Part model, mm, in its own coordinate system. A direction names the side the tool comes from. Round coordinates to 2 decimals unless told otherwise and drop trailing zeros. Loops run counter-clockwise (first coordinate to the right, second up) from the corner with the lowest first, then second, coordinate; pieces in that order, holes last. Notation, with made-up numbers: (53, -17.75) -> (109, -17.75) arc R13 ccw to (109, -6.75) -> close; hole circle Ø1 at (7, 76.25). An arc over 180 degrees is marked (long way). Use a Markdown table: item, result. Add a question column.
Item 1: Cut at A-A, the plane x = -10.5. List the corners of the cut face in (y, z), plus the area to 4 significant figures.
Item 2: Flat gauge pins, fed straight in: pin 1 (8 mm diameter, centred on x = -3.5, y = 23.5, fed in from -Z); pin 2 (0.6 mm diameter, centred on y = 13.5, z = 0.5, fed in from -X); pin 3 (6.5 mm diameter, centred on x = 16.5, y = -21.5, fed in from -Z). Where does each tip first touch, or does it go through?
Item 3: Two-plate mould, pull along Y, no slides. Class faces 4 (the face through (1, 49.682, -28)), 5 (the face through (48.16, -21.99, -3.94)), 6 (the face through (17, -22, -8)): pulls with the +Y half, pulls with the -Y half, needs draft (parallel to the pull), parting line crosses it, or undercut.
Item 4: Cut at B-B, the plane y = 37.5. List the corners of the cut face in (x, z), plus the area to 3 significant figures.
Item 5: Cut at C-C, the plane z = -2.5. List the corners of the cut face in (x, y).
Item 6: Which spindle directions (+Z, -Z, +X, -X, +Y, -Y) get a long thin tool onto all of the face, cutting with end or side? Do faces 1 (the face through (52, -22, -8)), 2 (the face through (1, 5, 2.54)), 3 (the face through (17.77, -24.39, -3.94)). Say none if no direction does.
Item 7: Cut at D-D, the plane x = 46.5. List the corners of the cut face in (y, z), plus the area to 3 significant figures.
Item 8: Probe line 1 (Y direction, x = -48, z = -0.5); line 2 (Z direction, x = 71, y = 17.5); line 3 (Z direction, x = 49, y = -20.5). List the from-to ranges inside material, lowest first. Write a range as [from, to].
```python
from build123d import *

# Parameters (mm, degrees)
SKETCH1_W           = 150
SKETCH1_H           = 85
BOSS_EXTRUDE1_DEPTH = 2.54
SKETCH2_W           = 20
SKETCH2_H           = 20
CUT_EXTRUDE1_DEPTH  = 2.54
SKETCH3_R           = 3
BOSS_EXTRUDE2_DEPTH = 8
SKETCH9_R           = 0.5
CUT_EXTRUDE7_DEPTH  = 4
CUT_EXTRUDE8_DEPTH  = 85
SKETCH11_W          = 150
SKETCH11_H          = 60
BOSS_EXTRUDE3_DEPTH = 2.54


with BuildPart() as part:
    # Sketch1 → Boss-Extrude1 (new body)
    with BuildSketch(Plane.XY):
        with Locations((2.158007809, 4.641833841)):
            Rectangle(SKETCH1_W, SKETCH1_H)
    extrude(amount=BOSS_EXTRUDE1_DEPTH)

    # Sketch2 → Cut-Extrude1 (cut)
    with BuildSketch(Plane(origin=(0, 0, 0), x_dir=(-1, 0, 0), z_dir=(0, 0, -1))):
        with Locations((7.841992191, -13.158166159)):
            Rectangle(SKETCH2_W, SKETCH2_H)
    extrude(amount=-CUT_EXTRUDE1_DEPTH, mode=Mode.SUBTRACT)

    # Sketch3 → Boss-Extrude2 (add)
    with BuildSketch(Plane(origin=(0, 0, 0), x_dir=(-1, 0, 0), z_dir=(0, 0, -1))):
        with Locations(Location((-51.158007809, -21.858166159, 0), (0, 0, 180))):
            Circle(SKETCH3_R)
        with Locations(Location((-16.158007809, -21.858166159, 0), (0, 0, 180))):
            Circle(SKETCH3_R)
    extrude(amount=BOSS_EXTRUDE2_DEPTH)

    # Sketch9 → Cut-Extrude7 (cut)
    with BuildSketch(Plane(origin=(0, 0, -8), x_dir=(-1, 0, 0), z_dir=(0, 0, -1))):
        with Locations((-51.158007809, -21.858166159)):
            Circle(SKETCH9_R)
        with Locations((-16.158007809, -21.858166159)):
            Circle(SKETCH9_R)
    extrude(amount=-CUT_EXTRUDE7_DEPTH, mode=Mode.SUBTRACT)

    # Sketch10 → Cut-Extrude8 (cut)
    with BuildSketch(Plane(origin=(0, 47.141833841, 0), x_dir=(1, 0, 0), z_dir=(0, 1, 0))):
        Polygon((-69.666992191, -1.27), (-69.666992191, -2.54), (-72.841992191, -2.54), (-72.841992191, 0), (-70.936992191, 0), (-70.936992191, -1.27), align=None)
        Polygon((75.888007809, 0), (75.888007809, -1.27), (74.618007809, -1.27), (74.618007809, -2.54), (77.158007809, -2.54), (77.158007809, 0), align=None)
    extrude(amount=-CUT_EXTRUDE8_DEPTH, mode=Mode.SUBTRACT)

    # Sketch11 → Boss-Extrude3 (add)
    with BuildSketch(Plane(origin=(0, 47.141833841, 0), x_dir=(1, 0, 0), z_dir=(0, 1, 0))):
        with Locations((2.158007809, 27.46)):
            Rectangle(SKETCH11_W, SKETCH11_H)
    extrude(amount=BOSS_EXTRUDE3_DEPTH)


solid = part.part
```
A:
| question | item | result |
|---|---|---|
| 1 | outline | (-37.86, 0) -> (-23.16, 0) -> (-23.16, 2.54) -> (-37.86, 2.54) -> close; (-3.16, 0) -> (47.14, 0) -> (47.14, -57.46) -> (49.68, -57.46) -> (49.68, 2.54) -> (-3.16, 2.54) -> close |
| 1 | area | 317.5 mm^2 |
| 2 | pin 1 | stops at z = 0 |
| 2 | pin 2 | stops at x = -70.94 |
| 2 | pin 3 | stops at z = -8 |
| 3 | face 4 | pulls with the +Y half |
| 3 | face 5 | undercut |
| 3 | face 6 | needs draft |
| 4 | outline | (-70.94, 0) -> (75.89, 0) -> (75.89, 1.27) -> (74.62, 1.27) -> (74.62, 2.54) -> (-69.67, 2.54) -> (-69.67, 1.27) -> (-70.94, 1.27) -> close |
| 4 | area | 370 mm^2 |
| 5 | outline | (-72.84, 47.14) -> (77.16, 47.14) -> (77.16, 49.68) -> (-72.84, 49.68) -> close; circle Ø6 at (16.16, -21.86); circle Ø6 at (51.16, -21.86) |
| 6 | face 1 | -Z, +X, -X, -Y |
| 6 | face 2 | +Z, +X, -X, +Y, -Y |
| 6 | face 3 | -Z |
| 7 | outline | (-37.86, 0) -> (47.14, 0) -> (47.14, -57.46) -> (49.68, -57.46) -> (49.68, 2.54) -> (-37.86, 2.54) -> close |
| 7 | area | 368 mm^2 |
| 8 | line 1 | y = [47.14, 49.68] |
| 8 | line 2 | z = [0, 2.54] |
| 8 | line 3 | z = [-8, 2.54] |
